Here's how the part is built. I have some questions about the finished solid (model axes, mm). Round coordinates to 2 decimals unless told otherwise and drop trailing zeros. Order: outer loops, then holes, each group sorted by start corner. A loop starts at its lowest first (then second) coordinate and runs counter-clockwise, first axis right, second up. Notation, with made-up numbers: (53.5, 72) - (66.5, 72) arc R28 cw to (66.5, 99) - close; hole circle Ø3 at (-34, 89). An arc over 180 degrees is marked (long way). One line per item, written item: value.
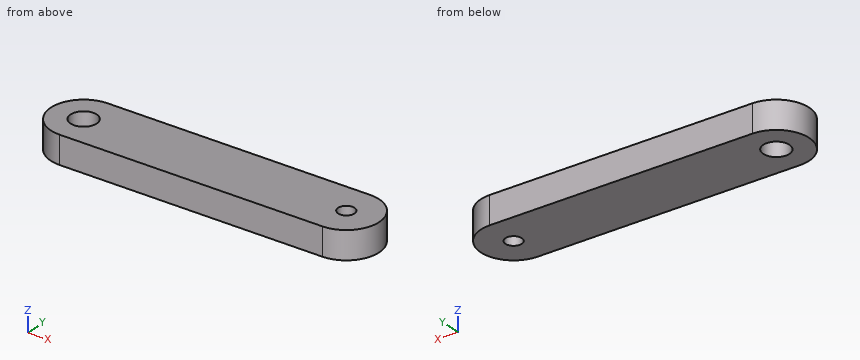
from build123d import *

# Parameters (mm, degrees)
SKETCH_1_R               = 2.5
EXTRUDE_1_DEPTH          = 8.5
CUT_EXTRUDE_2_DEPTH      = 91.95191037
CUT_EXTRUDE_2_DEPTH_BACK = 91.95191037
SKETCH_2_R               = 3.98703102


with BuildPart() as part:
    # 草图1 → 凸台-拉伸1 (new body)
    with BuildSketch(Plane.XY):
        with BuildLine():
            Line((0, 10), (80, 10))
            ThreePointArc((80, 10), (90, 0), (80, -10))
            Line((80, -10), (0, -10))
            ThreePointArc((0, -10), (-10, 0), (0, 10))
        make_face()
        Circle(SKETCH_1_R, mode=Mode.SUBTRACT)
        with Locations(Location((80, 0, 0), (0, 0, 180))):
            Circle(SKETCH_1_R, mode=Mode.SUBTRACT)
    extrude(amount=EXTRUDE_1_DEPTH)

    # 草图2 → 切除-拉伸2 (cut, two sides: drawn at the far end of the back side and taken through both)
    with BuildSketch(Plane.XY.offset(8.5).offset(-CUT_EXTRUDE_2_DEPTH_BACK)):
        Circle(SKETCH_2_R)
    extrude(amount=CUT_EXTRUDE_2_DEPTH + CUT_EXTRUDE_2_DEPTH_BACK, mode=Mode.SUBTRACT)


solid = part.part
Q1. If we section it at A-A, the plane y = 0: Please give me the cut outline in (x, z).
Results list:
outline: (-10, 0) - (-3.99, 0) - (-3.99, 8.5) - (-10, 8.5) - close; (3.99, 0) - (77.5, 0) - (77.5, 8.5) - (3.99, 8.5) - close; (82.5, 0) - (90, 0) - (90, 8.5) - (82.5, 8.5) - close
Q2. If we section it at D-D, the plane y = -6.5: Please give me the cut outline in (x, z).
Results list:
outline: (-7.6, 0) - (87.6, 0) - (87.6, 8.5) - (-7.6, 8.5) - close
Q3. If I drill on line 1 along X through (y, z) = (0.25, 5.25); line 2 along Y through (x, z) = (80, 6.25); line 3 along X through (y, z) = (-1.25, 3.25), over which ranges is the centre line in solid material (lowest first)?
Results list:
line 1: -10 to -3.98, 3.98 to 77.51, 82.49 to 90
line 2: -10 to -2.5, 2.5 to 10
line 3: -9.92 to -3.79, 3.79 to 77.83, 82.17 to 89.92
Q4. If we section it at C-C, the plane x = 79: Please give me the cut outline in (y, z).
Results list:
outline: (-10, 0) - (-2.29, 0) - (-2.29, 8.5) - (-10, 8.5) - close; (2.29, 0) - (10, 0) - (10, 8.5) - (2.29, 8.5) - close
Q5. If we section it at B-B, the plane z = 2.5: Please give me the cut outline in (x, y), then the cut area to 3 significant figures.
Results list:
outline: (0, -10) - (80, -10) arc R10 ccw to (80, 10) - (0, 10) arc R10 ccw to start; hole circle Ø7.97 at (0, 0); hole circle Ø5 at (80, 0)
area: 1,840 mm²
Q6. Will these pins go through, and if not, where does the flat tip stop? pin 1 (1.5 mm diameter, centred on y = 3.5, z = 1, fed in from +X); pin 2 (4 mm diameter, centred on x = 80, y = 0, fed in from +Z).
Results list:
pin 1: x = 89.61
pin 2: through
